Drawing for the job (mm, zero at the part's lowest x, y, z). A direction names the side the tool comes from. Give positions to 0.01 mm unless a question says otherwise; leave off trailing zeros. Loops run counter-clockwise (first coordinate to the right, second up) from the corner with the lowest first, then second, coordinate; pieces in that order, holes last.
1) Band-saw the part on B-B on x = 2.1. List the corners of the cut face in (y, z) (3 decimals).
2) Band-saw the part on C-C on y = 3. List the corners of the cut face in (x, z) (3 decimals), then the cut area to 3 significant figures.
3) Two-plate mould, pull along Y, no slides. Class the marked faces 1, 2, 3 and 4: +Y half, -Y half, draft (parallel to the pull), parting line (faces both ways), or undercut.
4) Wall check: line 1 (Y direction, x = 3, z = 6.75); line 2 (X direction, y = 4.95, z = 18.5). Give the ranges that are in metal, low to high.
5) Band-saw the part on A-A on z = 9.5. List the corners of the cut face in (x, y), then the cut area to 3 significant figures.
6) 3-axis set-ups, long thin cutter, end or side, ignore diameter. For the marked faces 5, 6 and 7: which of +Z, -Z, +X, -X, +Y, -Y reach the whole face in a straight line?
7) Flat gauge pins, fed straight in: P1, Ø2.5, axis at y = 2.5, z = 19, coming from the +X side; P2, Ø1.5, axis at x = 3, z = 6.5, coming from the +Y side; P3, Ø1.5, axis at y = 2.5, z = 6, coming from the +X side. Where does each tip first touch, or does it go through?
8) Band-saw the part on D-D on z = 17.75. List the corners of the cut face in (x, y).
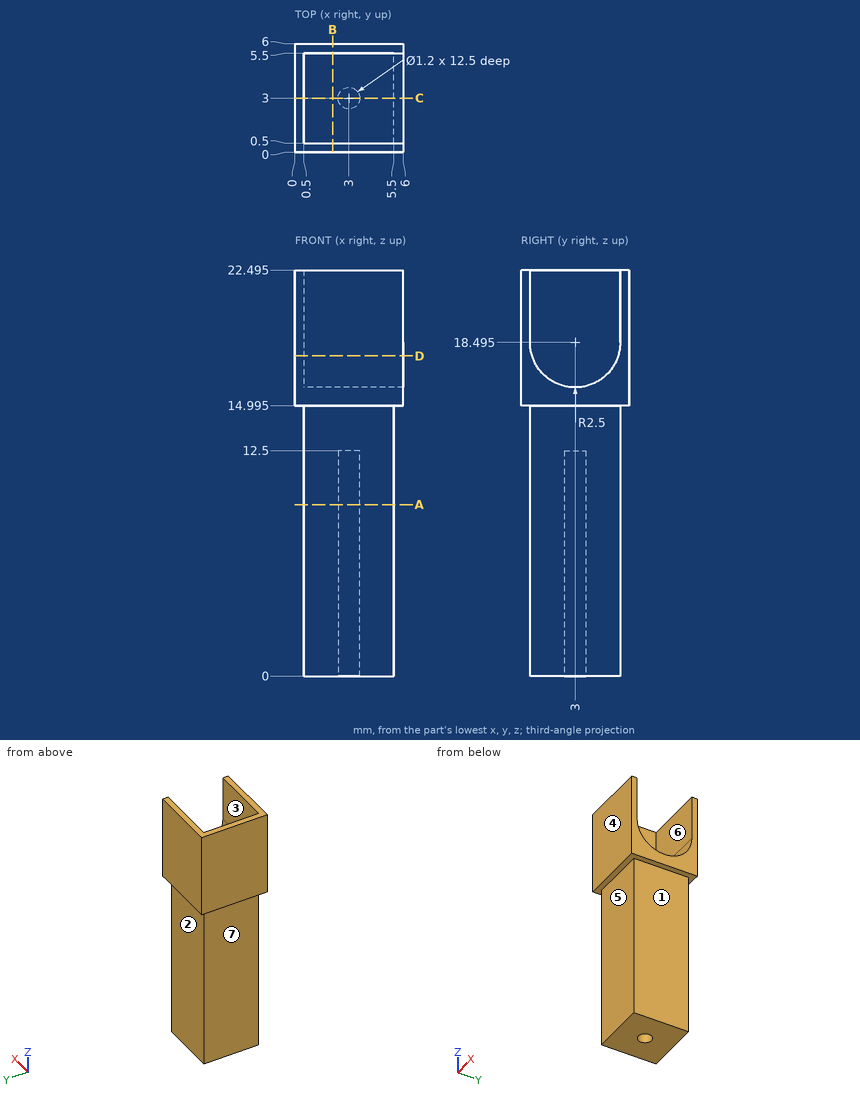
Findings below:
1. outline: (0, 14.995) - (0.5, 14.995) - (0.5, 0) - (5.5, 0) - (5.5, 14.995) - (6, 14.995) - (6, 22.495) - (5.5, 22.495) - (5.5, 18.495) arc R2.5 cw to (0.5, 18.495) - (0.5, 22.495) - (0, 22.495) - close
2. outline: (0, 14.995) - (0.5, 14.995) - (0.5, 0) - (2.4, 0) - (2.4, 12.5) - (3.6, 12.5) - (3.6, 0) - (5.5, 0) - (5.5, 14.995) - (6, 14.995) - (6, 15.995) - (0.5, 15.995) - (0.5, 22.495) - (0, 22.495) - close
2. area: 69.2 mm2
3. face 1: draft
3. face 2: +Y half
3. face 3: undercut
3. face 4: -Y half
4. line 1: y = 0.5 to 2.4, 3.6 to 5.5
4. line 2: x = 0 to 0.5
5. outline: (0.5, 0.5) - (5.5, 0.5) - (5.5, 5.5) - (0.5, 5.5) - close; hole circle Ø1.2 at (3, 3)
5. area: 23.9 mm2
6. face 5: -Z, +X, -X, -Y
6. face 6: +Z, +X
6. face 7: -Z, -X, +Y, -Y
7. P1: stops at x = 0.5
7. P2: stops at y = 5.5
7. P3: stops at x = 5.5
8. outline: (0, 0) - (6, 0) - (6, 0.61) - (0.5, 0.61) - (0.5, 5.39) - (6, 5.39) - (6, 6) - (0, 6) - close
